Design review of the part built by this model. Coordinates are the model's own, in mm. Face numbers are marked on the shaded views. A direction names the side the tool comes from. Round coordinates to 2 decimals unless told otherwise and drop trailing zeros. Loops run counter-clockwise (first coordinate to the right, second up) from the corner with the lowest first, then second, coordinate; pieces in that order, holes last. Notation, with made-up numbers: (85, 54) - (137, 54) arc R22 ccw to (137, 86) - close; hole circle Ø2 at (11.5, 44). An arc over 180 degrees is marked (long way). Return JSON: item names as keys, results as strings. Group by question number.
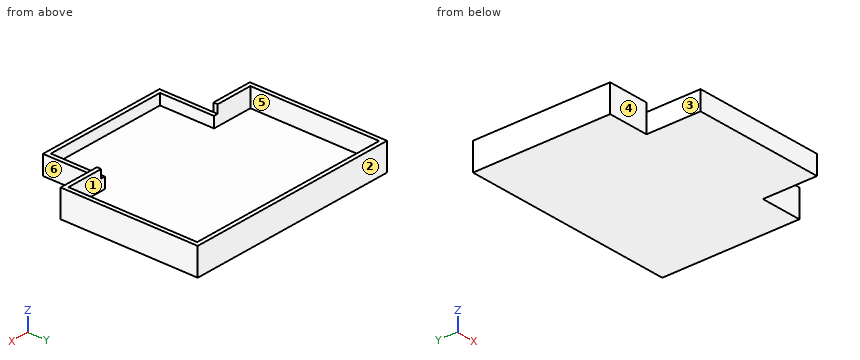
from build123d import *

# Parameters (mm, degrees)
PAD_DEPTH    = 1
PAD001_DEPTH = 1.3
PAD002_DEPTH = 1


with BuildPart() as part:
    # Sketch → Pad (new body)
    with BuildSketch(Plane.XY):
        Polygon((-13, 11.5), (13, 11.5), (13, -5), (8, -5), (8, -11.5), (-8, -11.5), (-8, -5), (-13, -5), align=None)
    extrude(amount=PAD_DEPTH)

    # Sketch001 (on DatumPlane) → Pad001 (join)
    with BuildSketch(Plane.XY.offset(1)):
        Polygon((-13, 11.5), (13, 11.5), (13, -5), (8, -5), (8, -11.5), (-8, -11.5), (-8, -5), (-13, -5), align=None)
        Polygon((-12.5, 11), (-12.5, -4.5), (-7.5, -4.5), (-7.5, -11), (7.5, -11), (7.5, -4.5), (12.5, -4.5), (12.5, 11), align=None, mode=Mode.SUBTRACT)
    extrude(amount=PAD001_DEPTH)

    # Sketch002 (on Face13 of Pad001) → Pad002 (join)
    with BuildSketch(Plane.XY.offset(2.3)):
        Polygon((-13, 11.5), (13, 11.5), (13, -5), (8, -5), (8, -4.5), (12.5, -4.5), (12.5, 11), (-12.5, 11), (-12.5, -4.5), (-8, -4.5), (-8, -5), (-13, -5), align=None)
    extrude(amount=PAD002_DEPTH)


solid = part.part
Q1. For line 1 (Y direction, x = 10, z = 2.1); line 2 (X direction, y = 8.5, z = 1.2); line 3 (X direction, y = -6, z = 2.1), list the stretches that pass through material, from the lowest coordinate up.
Q2. Add section B-B, the plane x = 5.25. State the section outline as (y, z) points, plus the area to 3 significant figures.
Q3. Add section A-A, the plane z = 1.6. State the section outline as (x, y) points.
Q4. Tool access review of the marked faces 4, 5 and 6: name each direction out of +Z, -Z, +X, -X, +Y, -Y from which nothing blocks a thin tool from reaching the whole face with its end or side.
Q5. Add section C-C, the plane y = 5. State the section outline as (x, z) points.
Q6. Draft analysis for pull direction X (two halves, no side actions). For the marked faces 1, 2 and 3, state which applies: pulls with the +X half, pulls with the -X half, needs draft (parallel to the pull), parting line crosses it, or undercut.
Q7. Insertion check: pin 1 Ø1 at (x, z) = (-10, 2) entering from -Y; pin 2 Ø12 at (x, y) = (7, -4.5) entering from -Z; pin 3 Ø1.5 at (x, y) = (-6.5, 4) entering from +Z; pin 4 Ø1.8 at (y, z) = (-7, 1) entering from +X. Each pin has a flat end and moves straight along its axis. Give the tip position at first contact, or say it passes through.
Evaluation:
{
 "1": {"line 1": "-5 to -4.5, 11 to 11.5", "line 2": "-13 to -12.5, 12.5 to 13", "line 3": "-8 to -7.5, 7.5 to 8"},
 "2": {"outline": "(-11.5, 0) - (11.5, 0) - (11.5, 3.3) - (11, 3.3) - (11, 1) - (-11, 1) - (-11, 2.3) - (-11.5, 2.3) - close", "area": "24.8 mm²"},
 "3": {"outline": "(-13, -5) - (-8, -5) - (-8, -11.5) - (8, -11.5) - (8, -5) - (13, -5) - (13, 11.5) - (-13, 11.5) - close; hole (-12.5, -4.5) - (-7.5, -4.5) - (-7.5, -11) - (7.5, -11) - (7.5, -4.5) - (12.5, -4.5) - (12.5, 11) - (-12.5, 11) - close"},
 "4": {"face 4": "+Z, -Z, -X, -Y", "face 5": "+Z", "face 6": "+Z, -Z, +X, -Y"},
 "5": {"outline": "(-13, 0) - (13, 0) - (13, 3.3) - (12.5, 3.3) - (12.5, 1) - (-12.5, 1) - (-12.5, 3.3) - (-13, 3.3) - close"},
 "6": {"face 1": "undercut", "face 2": "needs draft", "face 3": "pulls with the -X half"},
 "7": {"pin 1": "y = -5", "pin 2": "z = 0", "pin 3": "z = 1", "pin 4": "x = 8"}
}
